Check sheet for the modelled part. Datum: model origin and axes. Units: mm. Face numbers are marked on the shaded views. A direction names the side the tool comes from. Give positions to 0.01 mm unless a question says otherwise; leave off trailing zeros. Write each loop counter-clockwise with the first axis right and the second up, starting at its lowest first coordinate (ties: lowest second). Pieces come first, ordered by that corner, then holes. Notation, with made-up numbers: (-21, -30) -> (5, -30) arc R18 ccw to (5, -3) -> close; hole circle Ø1 at (-3, 33). An arc over 180 degrees is marked (long way). Answer as a JSON object with one key per item and string values.
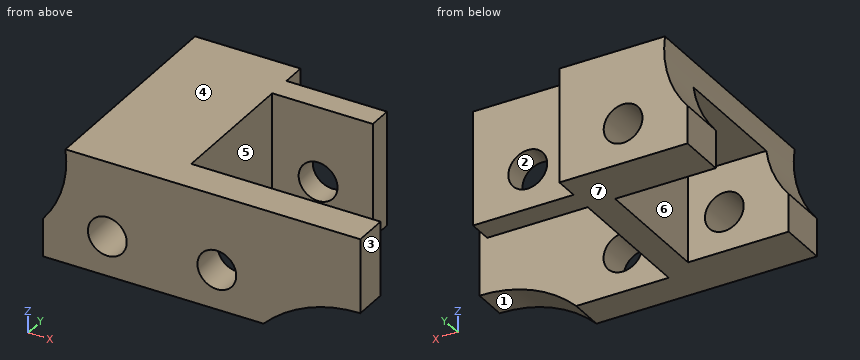
Autodesk Inventor part; units mm, degrees
ref_plane "YZ Plane" through (0, 0, 0) normal (1, 0, 0) x (0, 1, 0)
ref_plane "XZ Plane" through (0, 0, 0) normal (0, 1, 0) x (-1, 0, 0)
ref_plane "XY Plane" through (0, 0, 0) normal (0, 0, 1) x (1, 0, 0)
sketch "Sketch1" plane through (0, 0, 0) normal (0, 1, 0) x (-1, 0, 0)
  arc A0 (-17.5636, 5.8132) -> (-8.5833, 9.5329) centre (-17.5636, 18.5132) ccw
  arc A1 (-17.5636, 5.8132) -> (-8.5833, 9.5329) centre (-17.5636, 18.5132) ccw
  arc A2 (-8.5833, -9.3366) -> (-17.5636, -5.6168) centre (-17.5636, -18.3168) ccw
  arc A3 (-8.5833, -9.3366) -> (-17.5636, -5.6168) centre (-17.5636, -18.3168) ccw
  line L0 (-17.5636, 5.8132) -> (-17.5636, -5.6168)
  line L1 (-8.5833, 9.5329) -> (11.8765, 9.5329)
  line L2 (-8.5833, -9.3366) -> (11.1934, -9.3366)
  arc A4 (11.8765, 6.0101) -> (11.8765, -5.8137) centre (18.8929, 0.0982) ccw
  line L3 (11.8765, -9.3366) -> (11.1934, -9.3366)
  line L4 (11.8765, 9.5329) -> (11.8765, 6.0101)
  line L5 (11.8765, -5.8137) -> (11.8765, -9.3366)
  circle A5 centre (5.9079, 5.8536) radius 1.8
  circle A6 centre (5.9079, 5.8536) radius 1.8
  circle A7 centre (-4.2521, 5.8536) radius 1.8
  circle A8 centre (-4.2521, 5.8536) radius 1.8
  circle A9 centre (5.9079, -5.6573) radius 1.8
  circle A10 centre (5.9079, -5.6573) radius 1.8
  circle A11 centre (-4.2521, -5.6573) radius 1.8
  circle A12 centre (-4.2521, -5.6573) radius 1.8
  point P0 (12.4052, 6.5859)
extrude "Extrusion1" add sketch "Sketch1" along normal blind 4.445
sketch "Sketch2" plane through (0, 4.445, 0) normal (0, 1, 0) x (1, 0, 0)
  line L0 (-11.8765, -9.5329) -> (8.5833, -9.5329)
  line L1 (8.5833, 9.3366) -> (-11.8765, 9.3366)
  line L2 (0, -9.5329) -> (-2.54, -9.5329)
  line L3 (-2.54, 9.3366) -> (0, 9.3366)
  line L4 (0, 9.3366) -> (0, -9.5329)
  line L5 (-2.54, -1.3682) -> (-9.8062, -1.3682)
  line L6 (-2.54, 1.1718) -> (-9.8062, 1.1718)
  arc A0 (-11.8765, -6.0101) -> (-11.8765, 5.8137) centre (-18.8929, -0.0982) ccw
  arc A1 (-9.8062, -1.3682) -> (-9.8062, 1.1718) centre (-18.8929, -0.0982) ccw
  line L7 (-2.54, -9.5329) -> (-2.54, -1.3682)
  line L8 (-2.54, 1.1718) -> (-2.54, 9.3366)
  point P0 (0, 0)
  dimension "d2" = 2.54
extrude "Extrusion2" add sketch "Sketch2" along normal blind 11.43
sketch "Sketch3" plane through (0, 4.445, 0) normal (0, 1, 0) x (1, 0, 0)
  line L0 (0, -11.1934) -> (18.2988, -11.1934)
  line L1 (18.2988, -11.1934) -> (18.2988, 11.7125)
  line L2 (18.2988, 11.7125) -> (0, 11.7125)
  line L3 (0, 11.7125) -> (0, -11.1934)
  point P0 (0, 0)
extrude "Extrusion3" cut sketch "Sketch3" against normal blind 1.27
sketch "Sketch4" plane through (0, 15.875, 0) normal (0, 1, 0) x (1, 0, 0)
  arc A0 (20.271, 9.3366) -> (20.3081, -9.5329) centre (70.2056, 0) ccw
  line L0 (8.5833, -9.5329) -> (0, -9.5329)
  line L1 (-11.8765, -6.0101) -> (-11.8765, -9.5329)
  line L2 (7.4252, -9.5329) -> (-11.8765, -9.5329)
  line L3 (-11.8765, -9.5329) -> (-11.8765, -6.0101)
  arc A1 (-11.8765, -6.0101) -> (-11.8765, 5.8137) centre (-18.8929, -0.0982) ccw
  line L4 (-11.8765, 9.3366) -> (-11.8765, 5.8137)
  line L5 (-11.8765, 5.8137) -> (-11.8765, 9.3366)
  line L6 (-11.8765, 9.3366) -> (7.3957, 9.3366)
  line L7 (0, 9.3366) -> (8.5833, 9.3366)
  arc A2 (-11.8765, -6.0101) -> (-11.8765, 5.8137) centre (-18.8929, -0.0982) ccw
  line L8 (-11.8765, -9.5329) -> (8.5833, -9.5329)
  line L9 (-11.8765, -9.5329) -> (20.3081, -9.5329)
  line L10 (8.5833, 9.3366) -> (-11.8765, 9.3366)
  line L11 (-11.8765, 9.3366) -> (20.271, 9.3366)
  circle A3 centre (-5.9079, -5.8536) radius 1.8
  circle A4 centre (-5.9079, -5.8536) radius 1.8
  circle A5 centre (-5.9079, 5.6573) radius 1.8
  circle A6 centre (-5.9079, 5.6573) radius 1.8
  circle A7 centre (4.2521, -5.8536) radius 1.8
  circle A8 centre (4.2521, -5.8536) radius 1.8
  circle A9 centre (4.2521, 5.6573) radius 1.8
  circle A10 centre (4.2521, 5.6573) radius 1.8
  circle A11 centre (14.4121, -0.0982) radius 1.8
  point P0 (0, 0)
  dimension "d10" = 101.6
  dimension "d13" = 3.6
extrude "Extrusion4" add sketch "Sketch4" along normal blind 4.445
sketch "Sketch5" plane through (0, 20.32, 0) normal (0, 1, 0) x (1, 0, 0)
  line L0 (0, -9.5329) -> (20.3081, -9.5329)
  line L1 (20.3081, -9.5329) -> (0, -9.5329)
  line L2 (0, -9.5329) -> (0, 9.3366)
  line L3 (0, -9.5329) -> (0, 9.3366)
  line L4 (20.271, 9.3366) -> (0, 9.3366)
  line L5 (0, 9.3366) -> (20.271, 9.3366)
  arc A0 (20.271, 9.3366) -> (20.3081, -9.5329) centre (70.2056, 0) ccw
  circle A1 centre (4.2521, -5.8536) radius 1.8
  circle A2 centre (4.2521, -5.8536) radius 1.8
  circle A3 centre (4.2521, 5.6573) radius 1.8
  circle A4 centre (4.2521, 5.6573) radius 1.8
  circle A5 centre (14.4121, -0.0982) radius 1.8
  circle A6 centre (14.4121, -0.0982) radius 1.8
  point P0 (0, 0)
extrude "Extrusion5" cut sketch "Sketch5" against normal blind 2.2225
sketch "Sketch9" plane through (-11.8765, 0, 9.5329) normal (0, 0, 1) x (1, 0, 0)
  line L0 (-6.6056, 25.3261) -> (40.6741, 25.3261)
  line L1 (40.6741, 25.3261) -> (40.6741, -4.6288)
  line L2 (40.6741, -4.6288) -> (-6.6056, -4.6288)
  line L3 (-6.6056, -4.6288) -> (-6.6056, 25.3261)
  point P0 (11.8765, 0)
extrude "Extrusion7" cut sketch "Sketch9" against normal blind 8.255
sketch "Sketch10" plane through (0, 18.0975, 0) normal (0, 1, 0) x (1, 0, 0)
  circle A0 centre (4.2521, 5.6573) radius 1.8
  line L0 (0, -1.2779) -> (0, 9.3366)
  line L1 (9.3321, 9.9549) -> (21.2421, 9.9549)
  line L2 (21.2421, 9.9549) -> (21.2421, -3.3791)
  line L3 (21.2421, -3.3791) -> (9.3321, -3.3791)
  line L4 (9.3321, -3.3791) -> (9.3321, 9.9549)
  point P0 (0, 0)
extrude "Extrusion8" cut sketch "Sketch10" against normal blind 8.1534 contours L1 L2 L3 L4
properties part number "ServoBase"
1. Sectioned sample at B-B, the plane z = -5.25. State how many separate pieces and enclosed holes the cut face has, plus the area to 3 significant figures.
Determined:
{"separate pieces": "5", "enclosed holes": "0", "area": "157 mm^2"}
2. Scan lines: L1, parallel to Y at x = 4, z = -1.5 (1 decimal); L2, parallel to Y at x = -8.5, z = -5 (3 decimals); L3, parallel to X at y = 17, z = -7. Record each from-to range of solid material in increasing order. Write a range as [from, to].
Determined:
{"L1": "[0, 3.2], [15.9, 18.1]", "L2": "[0, 4.445], [15.875, 20.32]", "L3": "[-11.88, -7.11], [-4.71, 3.05], [5.45, 9.33]"}
3. Mould release check, pull along Z, two halves, no side actions. Record for the marked faces 1, 2, 3 and 4: released by +Z, released by -Z, zero draft, split by the parting line, or undercut.
Determined:
{"face 1": "released by -Z", "face 2": "undercut", "face 3": "zero draft", "face 4": "released by +Z"}
4. Sectioned sample at A-A, the plane x = 1. Enter the section's corners in (y, z) (1 decimal).
Determined:
{"outline": "(0, -9.3) -> (3.2, -9.3) -> (3.2, 1.3) -> (0, 1.3) -> close; (15.9, -9.3) -> (18.1, -9.3) -> (18.1, 1.3) -> (15.9, 1.3) -> close"}
5. Go/stop test with flat-tipped pins: P1, Ø4, axis at x = 4.25, z = -5.66, coming from the +Y side; P2, Ø1, axis at x = -3.5, y = 8, coming from the -Z side; P3, Ø1.1, axis at y = 16.5, z = -5, coming from the +X side. Record where each tip stops, or that it passes through.
Determined:
{"P1": "y = 18.1", "P2": "z = -1.17", "P3": "x = 9.33"}
6. Sectioned sample at D-D, the plane z = -1.5. Enter the section's corners in (x, y) (1 decimal).
Determined:
{"outline": "(-9.9, 0) -> (17.6, 0) -> (17.6, 3.2) -> (0, 3.2) -> (0, 15.9) -> (9.3, 15.9) -> (9.3, 18.1) -> (0, 18.1) -> (0, 20.3) -> (-9.9, 20.3) -> (-9.9, 15.9) -> (-2.5, 15.9) -> (-2.5, 4.4) -> (-9.9, 4.4) -> close"}
7. Sectioned sample at C-C, the plane x = -4.5. Enter the section's corners in (y, z) (3 decimals), plus the area to 3 significant figures.
Determined:
{"outline": "(0, -9.337) -> (4.445, -9.337) -> (4.445, -6.779) -> (0, -6.779) -> close; (0, -4.536) -> (4.445, -4.536) -> (4.445, -1.172) -> (15.875, -1.172) -> (15.875, -4.536) -> (20.32, -4.536) -> (20.32, 1.278) -> (0, 1.278) -> close; (15.875, -9.337) -> (20.32, -9.337) -> (20.32, -6.779) -> (15.875, -6.779) -> close", "area": "102 mm^2"}
8. Access from +Z, -Z, +X, -X, +Y, -Y to the whole of each face (thin tool, end or side, straight path). Record for the marked faces 5, 6 and 7.
Determined:
{"face 5": "+Z, -Z, +X", "face 6": "-Z, -X", "face 7": "-Z, +X, -X, +Y, -Y"}
